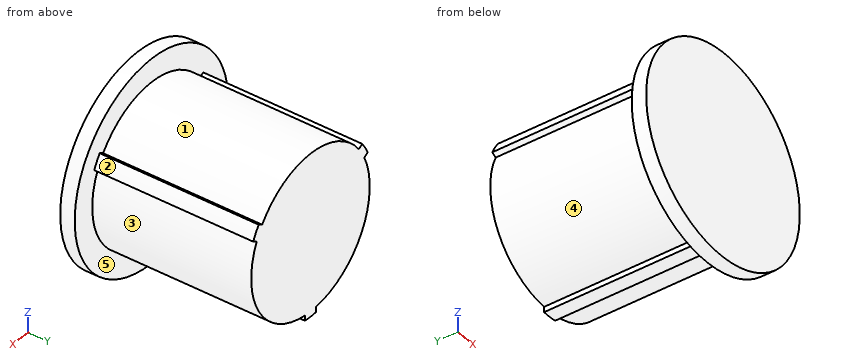
from build123d import *

# Parameters (mm, degrees)
BOSS_EXTRUDE1_DEPTH = 19.05
SKETCH6_W           = 0.608326788
SKETCH6_H           = 1.5875
SKETCH8_W           = 2.576826788
SKETCH8_H           = 1.5875


with BuildPart() as part:
    # Sketch1 → Boss-Extrude1 (new body)
    with BuildSketch(Plane(origin=(0, 0, 0), x_dir=(1, 0, 0), z_dir=(0, 1, 0))):
        with BuildLine():
            Line((-0.79375, 9.109483901), (-0.79375, 8.535673212))
            ThreePointArc((-0.79375, 8.535673212), (-7.424002774, 4.28625), (-7.78898484, -3.580428942))
            Line((-7.78898484, -3.580428942), (-8.285919473, -3.867334286))
            ThreePointArc((-8.285919473, -3.867334286), (-7.918936292, -4.572), (-7.492169473, -5.242149615))
            Line((-7.492169473, -5.242149615), (-6.99523484, -4.95524427))
            ThreePointArc((-6.99523484, -4.95524427), (0, -8.5725), (6.99523484, -4.95524427))
            Line((6.99523484, -4.95524427), (7.492169473, -5.242149615))
            ThreePointArc((7.492169473, -5.242149615), (7.918936292, -4.572), (8.285919473, -3.867334286))
            Line((8.285919473, -3.867334286), (7.78898484, -3.580428942))
            ThreePointArc((7.78898484, -3.580428942), (7.424002774, 4.28625), (0.79375, 8.535673212))
            Line((0.79375, 8.535673212), (0.79375, 9.109483901))
            ThreePointArc((0.79375, 9.109483901), (0, 9.144), (-0.79375, 9.109483901))
        make_face()
    extrude(amount=BOSS_EXTRUDE1_DEPTH)

    # Sketch6 → Cut-Revolve2 (revolve, cut)
    with BuildSketch(Plane(origin=(0, 0, 0), x_dir=(0, 0, -1), z_dir=(1, 0, 0))):
        with Locations((8.839836606, 0.79375)):
            Rectangle(SKETCH6_W, SKETCH6_H)
    revolve(axis=Axis((0, 19.730213777, 0), (0, -1, 0)), mode=Mode.SUBTRACT)

    # Sketch8 → Revolve2 (revolve)
    with BuildSketch(Plane(origin=(0, 0, 0), x_dir=(0, 0, -1), z_dir=(1, 0, 0))):
        with Locations((9.824086606, 0.79375)):
            Rectangle(SKETCH8_W, SKETCH8_H)
    revolve(axis=Axis((0, 4.48386458, 0), (0, -1, 0)))


solid = part.part
Read the model definition and answer for the solid it produces. Units are mm, in the model's axes. Face numbers are marked on the shaded views. A direction names the side the tool comes from. Coordinates: 2 decimals unless noted, no trailing zeros. Loops run counter-clockwise (first coordinate to the right, second up) from the corner with the lowest first, then second, coordinate; pieces in that order, holes last. Notation, with made-up numbers: (18.5, -16.5) -> (56.5, -16.5) arc R23 cw to (56.5, 9.5) -> close; hole circle Ø6 at (-2.75, -26.5). An arc over 180 degrees is marked (long way). Answer in a Markdown table with one row per item.
Item 1: A cutting plane is placed at D-D on x = -9. Determine the outline of the cut face in (y, z), plus the area to 3 significant figures.
Returned:
| item | result |
|---|---|
| outline | (0, -6.52) -> (1.59, -6.52) -> (1.59, 6.52) -> (0, 6.52) -> close |
| area | 20.7 mm^2 |
Item 2: Straight lines are drawn through the part: line 1 along Y through (x, z) = (10, -1.25); line 2 along Z through (x, y) = (0, 8.25); line 3 along Z through (x, y) = (5.25, 16.5). For each, find the intervals that lie inside material, in ascending order. Write a range as [from, to].
Returned:
| item | result |
|---|---|
| line 1 | y = [0, 1.59] |
| line 2 | z = [-9.14, 8.57] |
| line 3 | z = [-6.78, 6.78] |
Item 3: Each of these flat-tipped pins is pushed along its axis until it touches: P1, Ø1.5, axis at y = 6.5, z = -6, coming from the -X side; P2, Ø5, axis at x = -8.5, y = 9, coming from the -Z side; P3, Ø1, axis at y = 4.5, z = 6.5, coming from the +X side. Where does it stop, or does it pass through?
Returned:
| item | result |
|---|---|
| P1 | stops at x = -6.78 |
| P2 | stops at z = -6.12 |
| P3 | stops at x = 6.12 |
Item 4: A cutting plane is placed at C-C on y = 7.5. Determine the outline of the cut face in (x, z) (1 decimal), plus the area to 3 significant figures.
Returned:
| item | result |
|---|---|
| outline | (-8.3, 3.9) -> (-7.8, 3.6) arc R8.6 ccw to (-0.8, -8.5) -> (-0.8, -9.1) arc R9.1 ccw to (0.8, -9.1) -> (0.8, -8.5) arc R8.6 ccw to (7.8, 3.6) -> (8.3, 3.9) arc R9.1 ccw to (7.5, 5.2) -> (7, 5) arc R8.6 ccw to (-7, 5) -> (-7.5, 5.2) arc R9.1 ccw to start |
| area | 234 mm^2 |
Item 5: For the marked faces 1, 2, 3, 4 and 5, determine the directions among +Z, -Z, +X, -X, +Y, -Y from which every point of the face is accessible in a straight line to the end or side of a thin tool.
Returned:
| item | result |
|---|---|
| face 1 | +Z, +Y |
| face 2 | +Z, +X, +Y |
| face 3 | +X, +Y |
| face 4 | -X, +Y |
| face 5 | +Y |
Item 6: A cutting plane is placed at A-A on x = 0. Determine the outline of the cut face in (y, z).
Returned:
| item | result |
|---|---|
| outline | (0, -11.11) -> (1.59, -11.11) -> (1.59, -9.14) -> (19.05, -9.14) -> (19.05, 8.57) -> (1.59, 8.57) -> (1.59, 11.11) -> (0, 11.11) -> close |
Item 7: A cutting plane is placed at B-B on z = 0. Determine the outline of the cut face in (x, y).
Returned:
| item | result |
|---|---|
| outline | (-11.11, 0) -> (11.11, 0) -> (11.11, 1.59) -> (8.57, 1.59) -> (8.57, 19.05) -> (-8.57, 19.05) -> (-8.57, 1.59) -> (-11.11, 1.59) -> close |
